Can you work these out from the drawing? Everything is in mm from the part's minimum corner. Coordinates: 2 decimals unless noted, no trailing zeros. Write each loop counter-clockwise with the first axis right and the second up, starting at its lowest first coordinate (ties: lowest second). Pieces come first, ordered by that corner, then holes. Notation, with made-up numbers: (59, 36.5) - (89, 36.5) arc R20 ccw to (89, 73.5) - close; hole circle Ø8 at (68.25, -18). An arc over 180 degrees is marked (long way). One line per question, with ' | ' between items. Start each with the question number.
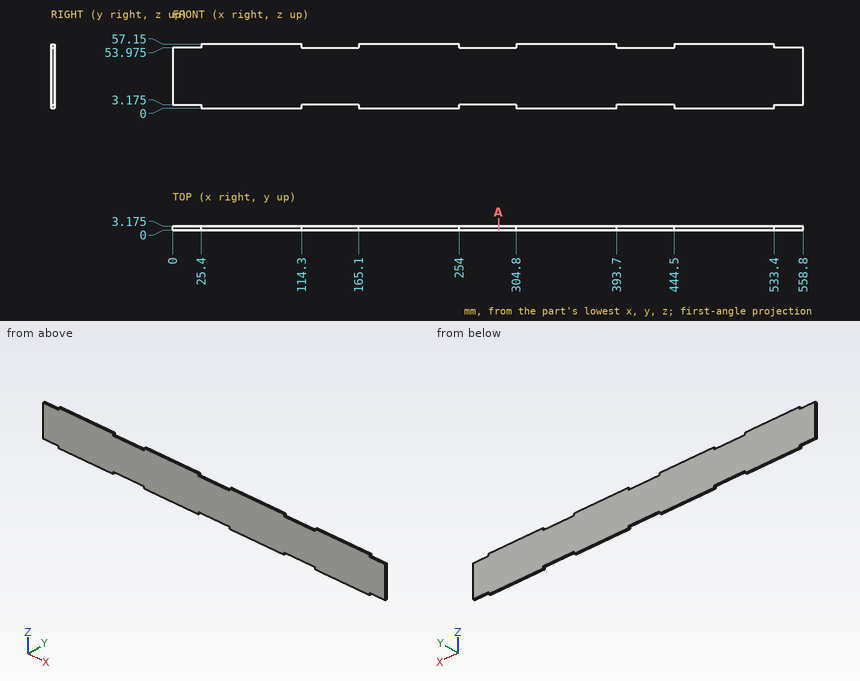
(1) If we section it at A-A on x = 289: List the corners of the cut face in (y, z) for me (3 decimals), plus the area to 3 significant figures.
(2) If I drill on probe 1 along Z at (x, y) = (401, 2.1) (3 decimals), over which ranges is the centre line in solid material (lowest first)?
(3) I'm going to push flat-ended pins straight in: pin 1 (1.6 mm diameter, centred on x = 146.5, y = 1.5, fed in from -Z) (3 decimals); pin 2 (1 mm diameter, centred on x = 8, y = 2, fed in from +Z) (3 decimals); pin 3 (1.6 mm diameter, centred on y = 2, z = 1, fed in from -X). Where does each tip first touch, or does it pass through?
Values:
1) outline: (0, 3.175) - (3.175, 3.175) - (3.175, 53.975) - (0, 53.975) - close | area: 161 mm2
2) probe 1: 3.175 to 53.975
3) pin 1: z = 3.175 | pin 2: z = 53.975 | pin 3: x = 25.4
